from build123d import *

# Parameters (mm, degrees)
F0_R     = 5.1
F1_DEPTH = 45
F2_DEPTH = 2.5


with BuildPart() as f1:
    # F0 (on Top) → F1 (new body)
    with BuildSketch(Plane.XY):
        with BuildLine():
            Line((47.999931, -27.712773), (0, 0))
            Line((0, 0), (-47.425757, -27.381273))
            ThreePointArc((-47.425757, -27.381273), (-36.236956, -57.202053), (-35.533555, -89.045002))
            ThreePointArc((-35.533555, -89.045002), (-24.364362, -85.504329), (-17.5, -95))
            ThreePointArc((-17.5, -95), (-20.428932, -102.071068), (-27.5, -105))
            Line((-27.5, -105), (27.5, -105))
            ThreePointArc((27.5, -105), (19.686236, -88.7594), (37.252515, -92.789018))
            ThreePointArc((37.252515, -92.789018), (36.797234, -59.288231), (47.999931, -27.712773))
        make_face()
        with BuildLine():
            ThreePointArc((-17.5, -95), (-24.364362, -85.504329), (-35.533555, -89.045002))
            ThreePointArc((-35.533555, -89.045002), (-36.431685, -99.497223), (-27.5, -105))
            ThreePointArc((-27.5, -105), (-20.428932, -102.071068), (-17.5, -95))
        make_face()
        with BuildLine():
            ThreePointArc((-22.4, -95), (-23.893755, -98.606245), (-27.5, -100.1))
            ThreePointArc((-27.5, -100.1), (-31.106245, -91.393755), (-22.4, -95))
        make_face(mode=Mode.SUBTRACT)
        with BuildLine():
            ThreePointArc((37.5, -95), (37.437936, -93.887605), (37.252515, -92.789018))
            ThreePointArc((37.252515, -92.789018), (19.686236, -88.7594), (27.5, -105))
            ThreePointArc((27.5, -105), (34.571068, -102.071068), (37.5, -95))
        make_face()
        with Locations((27.5, -95)):
            Circle(F0_R, mode=Mode.SUBTRACT)
    extrude(amount=F1_DEPTH)

    # F0 (on Top) → F2 (join)
    with BuildSketch(Plane.XY):
        with Locations((27.5, -95)):
            Circle(F0_R)
        with BuildLine():
            ThreePointArc((-22.4, -95), (-31.106245, -91.393755), (-27.5, -100.1))
            ThreePointArc((-27.5, -100.1), (-23.893755, -98.606245), (-22.4, -95))
        make_face()
    extrude(amount=F2_DEPTH)


solid = f1.part
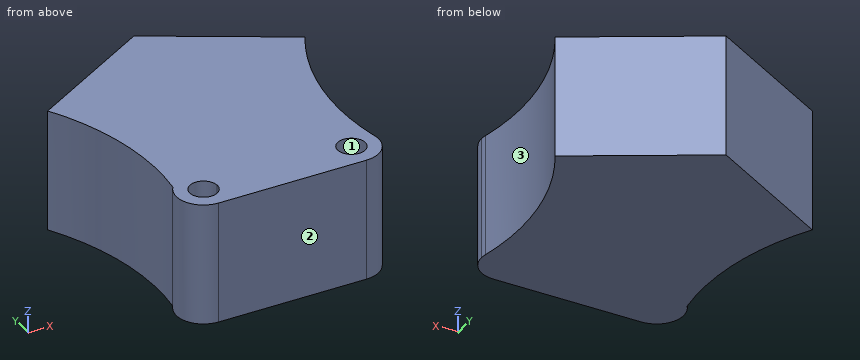
Design review of the part built by this model. Coordinates are the model's own, in mm. Face numbers are marked on the shaded views. Coordinates: 2 decimals unless noted, no trailing zeros. Order: outer loops, then holes, each group sorted by start corner. A loop starts at its lowest first (then second) coordinate and runs counter-clockwise, first axis right, second up. Notation, with made-up numbers: (84.5, 7.25) - (91.5, 7.25) arc R7 cw to (91.5, 11.25) - close; hole circle Ø2 at (19, 77.5). An arc over 180 degrees is marked (long way). Put each result on its own line as item: value.
1) The part is to be moulded in two halves that separate along X. For the marked faces 1, 2 and 3, say which applies: released by +X, released by -X, zero draft, split by the parting line, or undercut.
Response values:
face 1: undercut
face 2: zero draft
face 3: released by +X
2) Take a section at A-A, the plane z = 7.5. Give the boundary of the cut face in (x, y) (3 decimals).
Response values:
outline: (-47.426, -27.381) arc R95 cw to (-35.534, -89.045) arc R10 ccw to (-27.5, -105) - (27.5, -105) arc R10 ccw to (37.5, -95) arc R10 ccw to (37.253, -92.789) arc R95 cw to (48, -27.713) - (0, 0) - close; hole (-27.5, -100.1) arc R5.1 ccw to (-22.4, -95) arc R5.1 ccw (long way) to start; hole circle Ø10.2 at (27.5, -95)
3) Insertion check: P1, Ø1, axis at x = 21, z = 6.5, coming from the +Y side; P2, Ø3, axis at x = 29, y = -96, coming from the +Z side; P3, Ø8, axis at y = -52.5, z = 17, coming from the -X side. Each pin has a flat end and moves straight along its axis. Give the tip position at first contact, or say it passes through.
Response values:
P1: stops at y = -11.84
P2: stops at z = 2.5
P3: stops at x = -38.34
4) Take a section at D-D, the plane y = -33. Give the boundary of the cut face in (x, z).
Response values:
outline: (-44.4, 0) - (45.2, 0) - (45.2, 45) - (-44.4, 45) - close
5) Take a section at B-B, the plane y = -96.5. Give the boundary of the cut face in (x, z).
Response values:
outline: (-37.39, 0) - (37.39, 0) - (37.39, 45) - (32.37, 45) - (32.37, 2.5) - (22.63, 2.5) - (22.63, 45) - (-22.63, 45) - (-22.63, 2.5) - (-32.37, 2.5) - (-32.37, 45) - (-37.39, 45) - close
6) Take a section at C-C, the plane x = 5. Give the boundary of the cut face in (y, z).
Response values:
outline: (-105, 0) - (-2.89, 0) - (-2.89, 45) - (-105, 45) - close
7) Wall thickness on L1, parallel to X at y = -90.5, z = 35; L2, parallel to Z at x = -31, y = -97.5; L3, parallel to Y at x = -17.5, z = 35: over which ranges is each line inside the solid? List them lowest first. Write a range as from..to.
Response values:
L1: x = -36.43..-29.9, -25.1..25.1, 29.9..36.84
L2: z = 0..2.5
L3: y = -105..-10.1
